Design review of the part built by this model. Coordinates are the model's own, in mm. A direction names the side the tool comes from. Coordinates: 2 decimals unless noted, no trailing zeros. Write each loop counter-clockwise with the first axis right and the second up, starting at its lowest first coordinate (ties: lowest second). Pieces come first, ordered by that corner, then holes.
Q1. Take a section at A-A (y = 1.45). Give the boundary of the cut face in (x, z) (3 decimals), and give its area (3 significant figures).
Q2. Take a section at D-D (x = 0). Give the boundary of the cut face in (y, z) (3 decimals).
Q3. For probe 1 along X at (y, z) = (0.05, -7); probe 2 along Z at (x, y) = (5.5, 2) (3 decimals); probe 3 along X at (y, z) = (1.1, 6.75), list the stretches that pass through material, from the lowest coordinate up.
Q4. Take a section at B-B (x = -6). Give the boundary of the cut face in (y, z) (3 decimals).
Q5. Machinability: for faces 1 (the cylindrical face through (-0.132, -0.493, -2.915)), 2 (the flat face through (-6, 2, -6.25)), 3 (the flat face through (-0.9, 3, 7)), which of the approach directions +Z, -Z, +X, -X, +Y, -Y give a long, thin tool a straight path to every point of the face, cutting with its end or side? Answer none if there is none.
Q6. Mouldability with a two-part tool opening along Z and no side actions: class faces 4 (the flat face through (0, 0.2, 8)), 5 (the cylindrical face through (-6.25, 2.52, -0.12)) as pulls with the +Z half, pulls with the -Z half, needs draft (parallel to the pull), parting line crosses it, or undercut.
Q7. Insertion check: pin 1 (0.9 mm diameter, centred on y = 3, z = -6.5, fed in from +X); pin 2 (0.9 mm diameter, centred on x = 0.5, z = 9, fed in from +Y); pin 3 (0.9 mm diameter, centred on y = 1, z = -6.5, fed in from -X). Each pin has a flat end and moves straight along its axis. Give the tip position at first contact, or say it passes through.
Q8. Take a section at C-C (z = 0). Give the boundary of the cut face in (x, y), and give its area (3 significant figures).
Autodesk Inventor part; units mm, degrees
ref_plane "YZ Plane" through (0, 0, 0) normal (1, 0, 0) x (0, 1, 0)
ref_plane "XZ Plane" through (0, 0, 0) normal (0, 1, 0) x (-1, 0, 0)
ref_plane "XY Plane" through (0, 0, 0) normal (0, 0, 1) x (1, 0, 0)
sketch "Sketch1" plane through (0, 0, 0) normal (0, 1, 0) x (-1, 0, 0)
  arc A0 (4.1548, -6.25) -> (-4.1548, -6.25) centre (0, 0) ccw
  circle A1 centre (0, 0) radius 6.25 construction
  line L0 (-7, -6.25) -> (-7, -7.985)
  line L1 (-7, -7.985) -> (7, -7.985)
  line L2 (7, -7.985) -> (7, -6.25)
  line L3 (0, 7.505) -> (-2.894, 7.505)
  line L4 (7, -6.25) -> (4.1548, -6.25)
  line L5 (-4.1548, -6.25) -> (-7, -6.25)
  dimension "d0" = 15.01
  dimension "d1" = 12.5
  dimension "d2" = 15.49
  dimension "d4" = 14
  dimension "d5" = 7
extrude "Extrusion1" add sketch "Sketch1" along normal blind 4
sketch "Sketch2" plane through (0, 4, 0) normal (0, 1, 0) x (1, 0, 0)
  circle A0 centre (0, 0) radius 6.25
  line L0 (-0.9, -7.9572) -> (0.9, -7.9572)
  line L1 (0.9, -7.9572) -> (0.9, 8.949)
  line L2 (0.9, 8.949) -> (-0.9, 8.949)
  line L3 (-0.9, 8.949) -> (-0.9, -7.9572)
  dimension "d8" = 12.5
  dimension "d11" = 1.8
  dimension "d12" = 0.9
extrude "Extrusion2" cut sketch "Sketch2" against normal blind 3
sketch "Sketch3" plane through (0, 0, 0) normal (0, -1, 0) x (1, 0, 0)
  line L0 (0.9, 5.5692) -> (-0.9, 5.5692)
  line L1 (-0.9, 5.5692) -> (-0.9, 9.4)
  line L2 (-0.9, 9.4) -> (0.9, 9.4)
  line L3 (0.9, 9.4) -> (0.9, 5.5692)
  line L4 (-0.9, -6.2525) -> (0.9, -6.2525)
  line L5 (0.9, -6.2525) -> (0.9, -9.4)
  line L6 (0.9, -9.4) -> (-0.9, -9.4)
  line L7 (-0.9, -9.4) -> (-0.9, -6.2525)
  point P0 (0, 0)
  dimension "d13" = 1.8
  dimension "d14" = 1.8
  dimension "d15" = 0.9
  dimension "d16" = 0.9
  dimension "d17" = 18.8
  dimension "d18" = 9.4
extrude "Extrusion3" add sketch "Sketch3" against normal blind 0.2
sketch "Sketch4" plane through (0, 0, 0) normal (0, -1, 0) x (1, 0, 0)
  circle A0 centre (0, -3.51) radius 0.61
  circle A1 centre (0, 3.51) radius 0.455
  point P0 (0, 0)
  dimension "d21" = 3.51
  dimension "d22" = 3.51
  dimension "d23" = 1.22
  dimension "d24" = 0.91
extrude "Extrusion4" add sketch "Sketch4" along normal blind 1
properties part number "Keystone1056_12_5mmCoinCell"
Response:
1. outline: (-7, -7.985) - (-0.9, -7.985) - (-0.9, -6.185) arc R6.25 cw to (-0.9, 6.185) - (-0.9, 7.451) arc R7.505 ccw to (-4.155, -6.25) - (-7, -6.25) - close; (0.9, -7.985) - (7, -7.985) - (7, -6.25) - (4.155, -6.25) arc R7.505 ccw to (0.9, 7.451) - (0.9, 6.185) arc R6.25 cw to (0.9, -6.185) - close
1. area: 66.0 mm2
2. outline: (-1, -4.12) - (0, -4.12) - (0, -9.4) - (0.2, -9.4) - (0.2, -7.985) - (1, -7.985) - (1, 7.505) - (0.2, 7.505) - (0.2, 9.4) - (0, 9.4) - (0, 3.965) - (-1, 3.965) - (-1, 3.055) - (0, 3.055) - (0, -2.9) - (-1, -2.9) - close
3. probe 1: x = -7 to 7
3. probe 2: z = -7.985 to -6.25, -5.106 to -2.969, 2.969 to 5.106
3. probe 3: x = -3.28 to -0.9, 0.9 to 3.28
4. outline: (0, -7.985) - (4, -7.985) - (4, -6.25) - (0, -6.25) - close; (0, -4.508) - (4, -4.508) - (4, -1.75) - (1, -1.75) - (1, 1.75) - (4, 1.75) - (4, 4.508) - (0, 4.508) - close
5. face 1: -Y
5. face 2: -X, +Y, -Y
5. face 3: +Z, -Z, +Y
6. face 4: needs draft
6. face 5: undercut
7. pin 1: stops at x = 7
7. pin 2: stops at y = 0.2
7. pin 3: stops at x = -7
8. outline: (-7.5, 0) - (7.5, 0) - (7.5, 4) - (6.25, 4) - (6.25, 1) - (-6.25, 1) - (-6.25, 4) - (-7.5, 4) - close
8. area: 22.5 mm2
